Geometry: final body of the model. Coordinates: model frame, mm. Face numbers are marked on the shaded views. A direction names the side the tool comes from. Coordinates: 2 decimals unless noted, no trailing zeros. Write each loop counter-clockwise with the first axis right and the second up, starting at its lowest first coordinate (ties: lowest second). Pieces come first, ordered by that corner, then holes. Notation, with made-up numbers: (20.25, 69.25) -> (54.25, 69.25) arc R24 ccw to (54.25, 108.25) -> close; hole circle Ø5 at (21, -16). An arc over 180 degrees is marked (long way). One line per item, written item: value. Start each with the question number.
from build123d import *

# Parameters (mm, degrees)
REVOLUTION002_ANGLE       = -180
PAD017_DEPTH              = 0.4
BODY015_PLACEMENT_ANGLE   = 180
PAD016_DEPTH              = 2.4
FUSION003_PLACEMENT_ANGLE = 140


with BuildPart() as light002:
    # Sketch027 (on Face1 of ShapeBinder005) → Revolution002 (revolve)
    with BuildSketch(Plane.XY.offset(2.4)):
        with BuildLine():
            ThreePointArc((-2.75, 0), (0, -2.75), (2.75, 0))
            Line((-2.75, 0), (2.75, 0))
        make_face()
    revolve(axis=Axis((-2.75, 0, 2.4), (1, 0, 0)), revolution_arc=REVOLUTION002_ANGLE)


with BuildPart() as body015:
    # Sketch028 (on Face1 of ShapeBinder006) → Pad017 (new body)
    with BuildSketch(Plane(origin=(0, 0, 0), x_dir=(1, 0, 0), z_dir=(0, 0, -1))):
        with BuildLine():
            Line((3.65, 1.5), (6.65, 1.5))
            Line((6.65, 1.5), (6.65, 2))
            Line((6.65, 2), (8.65, 2))
            Line((8.65, 2), (8.65, 0.2))
            Line((8.65, 0.2), (6.65, 0.2))
            Line((6.65, 0.2), (6.65, 0.7))
            Line((6.65, 0.7), (4.45, 0.7))
            Line((4.45, 0.7), (4.45, -0.2))
            ThreePointArc((4.45, -0.2), (3.8, -0.85), (4.45, -1.5))
            Line((4.45, -1.5), (-6.65, -1.5))
            Line((-6.65, -1.5), (-6.65, -1.85))
            Line((-6.65, -1.85), (-8.65, -1.85))
            Line((-8.65, -1.85), (-8.65, -0.25))
            Line((-8.65, -0.25), (-6.65, -0.25))
            Line((-6.65, -0.25), (-6.65, -0.6))
            Line((-6.65, -0.6), (-4.95, -0.6))
            Line((-4.95, -0.6), (-4.95, 1.5))
            Line((-4.95, 1.5), (3.65, 1.5))
        make_face()
    extrude(amount=-PAD017_DEPTH)


with BuildPart() as body015_1:
    # Body015 placement: moved
    add(body015.part.moved(Location((0, 0, 1.4))).rotate(Axis((0, 0, 1.4), (1, 0, 0)), BODY015_PLACEMENT_ANGLE))


with BuildPart() as led3:
    # Sketch026 → Pad016 (new body)
    with BuildSketch(Plane.XY):
        with BuildLine():
            Line((-3.65, 1.75), (-3.65, -1.75))
            ThreePointArc((-3.65, -1.75), (0, -4), (3.65, -1.75))
            Line((3.65, 1.75), (3.65, -1.75))
            ThreePointArc((3.65, 1.75), (0, 4), (-3.65, 1.75))
        make_face()
    extrude(amount=PAD016_DEPTH)

    # Fusion003: union light002, Body015
    add(light002.part)
    add(body015_1.part)


with BuildPart() as led3_1:
    # Fusion003 placement: moved
    add(led3.part.moved(Location((-27, -36.5, -2.8))).rotate(Axis((-27, -36.5, -2.8), (0, 0, 1)), FUSION003_PLACEMENT_ANGLE))


solid = led3_1.part
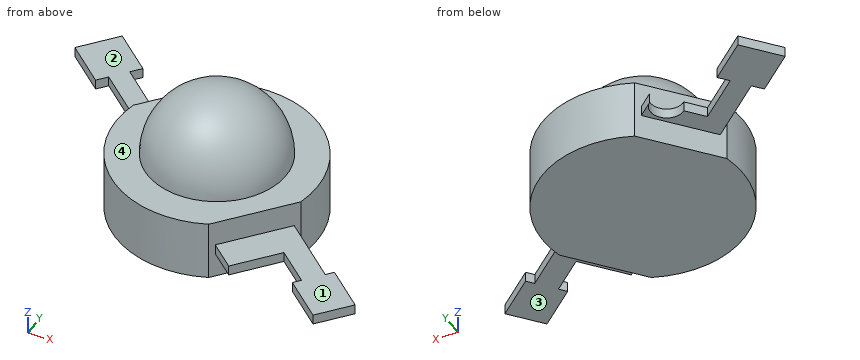
Q1. Cut plane C-C on y = -37.25. Output: boundary loops of the cut face in (x, z), and give its area (3 significant figures).
Q2. Line query: L1, parallel to Z at x = -24.75, y = -38.5; L2, parallel to Z at x = -22.25, y = -39; L3, parallel to X at y = -38.75, z = 0.6. Output: solid intervals per line, ascending. Write a range as from..to.
Q3. Cut plane A-A on x = -27.5. Output: boundary loops of the cut face in (y, z).
Q4. First-contact query: P1, Ø1.3, axis at x = -33.5, y = -34, coming from the -Z side; P2, Ø4.5, axis at x = -21.5, y = -39.5, coming from the +Z side; P3, Ø1, axis at x = -26, y = -32.5, coming from the +Z side. Flat tips, straight axial feed; report the tip coordinate or a pass-through.
Q5. Cut plane B-B on z = -2.05. Output: boundary loops of the cut face in (x, y) (3 decimals).
Q6. Access query for the marked faces 1, 2, 3 and 4. Directions: +Z, -Z, +X, -X, +Y, -Y. A direction counts if a zero-diameter tool reaches every point of the face in a straight line with its end or side. Return the directions, or none.
Q7. Cut plane D-D on y = -38.5. Output: boundary loops of the cut face in (x, z).
Solution:
1. outline: (-30.95, -2.8) -> (-23.03, -2.8) -> (-23.03, -0.4) -> (-24.35, -0.4) arc R2.65 ccw to (-29.65, -0.4) -> (-30.95, -0.4) -> close
1. area: 30.0 mm²
2. L1: -2.8..-0.4
2. L2: -1.8..-1.4
2. L3: -28.22..-25.78
3. outline: (-40.48, -2.8) -> (-32.5, -2.8) -> (-32.5, -0.4) -> (-33.8, -0.4) arc R2.7 ccw to (-39.2, -0.4) -> (-40.48, -0.4) -> close
4. P1: z = -1.8
4. P2: z = -1.4
4. P3: z = -0.4
5. outline: (-30.921, -35.494) arc R4.086 ccw to (-25.329, -40.187) -> (-23.079, -37.506) arc R4.086 ccw to (-28.671, -32.813) -> close
6. face 1: +Z, +X, -Y
6. face 2: +Z, -X, +Y
6. face 3: -Z, +X, -Y
6. face 4: +Z
7. outline: (-30.47, -2.8) -> (-23.91, -2.8) -> (-23.91, -1.8) -> (-22.28, -1.8) -> (-22.28, -1.4) -> (-23.91, -1.4) -> (-23.91, -0.4) -> (-25.11, -0.4) arc R1.89 ccw to (-28.89, -0.4) -> (-30.47, -0.4) -> close
